For this review, take the finished solid that the model builds, in its own axes (mm). Round coordinates to 2 decimals unless told otherwise and drop trailing zeros. Loops run counter-clockwise (first coordinate to the right, second up) from the corner with the lowest first, then second, coordinate; pieces in that order, holes last.
1. Consider section D-D on z = 77. State the section outline as (x, y) points.
2. Consider section C-C on y = -16.5. State the section outline as (x, z) points.
3. Consider section A-A on z = 11. State the section outline as (x, y) points (3 decimals).
4. Consider section B-B on y = -162.5. State the section outline as (x, z) points, then the cut area to 3 significant figures.
5. Clearance check with flat-ended pins moving along their axes: pin 1 Ø5 at (y, z) = (-46.5, 99) entering from -X; pin 2 Ø0.9 at (x, y) = (2, -185.5) entering from +Z; pin 3 Ø0.9 at (x, y) = (1, -186) entering from -Z; pin 4 Ø0.9 at (x, z) = (1, 190.5) entering from +Y. State where each tip first meets the part, or that it passes through.
6. To check wall thickness, follow line 1 along Z through (x, y) = (1.7, -150); line 2 along Z through (x, y) = (1.4, -176); line 3 along Z through (x, y) = (0.35, -10). State the ranges of each line that lie inside material, in increasing order.
Autodesk Inventor part; units mm, degrees
ref_plane "YZ Plane" through (0, 0, 0) normal (1, 0, 0) x (0, 1, 0)
ref_plane "XZ Plane" through (0, 0, 0) normal (0, 1, 0) x (-1, 0, 0)
ref_plane "XY Plane" through (0, 0, 0) normal (0, 0, 1) x (1, 0, 0)
sketch "Sketch1" plane through (0, 0, 0) normal (1, 0, 0) x (0, 1, 0)
  line L0 (3, 191.4188) -> (-194, 191.4188) construction
  line L1 (-194, 191.4188) -> (-194, -8.5812) construction
  line L2 (-194, -8.5812) -> (3, -8.5812) construction
  line L3 (3, -8.5812) -> (3, 191.4188) construction
  line L4 (0, 188.4188) -> (-191, 188.4188) construction
  line L5 (-191, 188.4188) -> (-191, -5.5812) construction
  line L6 (-191, -5.5812) -> (0, -5.5812) construction
  line L7 (0, -5.5812) -> (0, 188.4188) construction
  line L8 (-165.5, -5.5812) -> (-165.5, -8.5812) construction
  line L9 (-194, -5.5812) -> (-165.5, -5.5812)
  line L10 (-165.5, -5.5812) -> (-165.5, -8.5812)
  line L11 (-165.5, -8.5812) -> (-145.5, -8.5812)
  line L12 (-145.5, -8.5812) -> (-145.5, -5.5812)
  line L13 (-145.5, -5.5812) -> (-125.5, -5.5812)
  line L14 (-125.5, -5.5812) -> (-125.5, -8.5812)
  line L15 (3, -5.5812) -> (-25.5, -5.5812)
  line L16 (-25.5, -5.5812) -> (-25.5, -8.5812)
  line L17 (-25.5, -8.5812) -> (-45.5, -8.5812)
  line L18 (-45.5, -8.5812) -> (-45.5, -5.5812)
  line L19 (-45.5, -5.5812) -> (-65.5, -5.5812)
  line L20 (-65.5, -5.5812) -> (-65.5, -8.5812)
  line L21 (-65.5, -8.5812) -> (-85.5, -8.5812)
  line L22 (-85.5, -8.5812) -> (-85.5, -5.5812)
  line L23 (-85.5, -5.5812) -> (-105.5, -5.5812)
  line L24 (-105.5, -5.5812) -> (-105.5, -8.5812)
  line L25 (-105.5, -8.5812) -> (-125.5, -8.5812)
  line L26 (-194, 188.4188) -> (-165.5, 188.4188)
  line L27 (-165.5, 188.4188) -> (-165.5, 191.4188)
  line L28 (3, 188.4188) -> (-25.5, 188.4188)
  line L29 (-25.5, 188.4188) -> (-25.5, 191.4188)
  line L30 (-25.5, 191.4188) -> (-45.5, 191.4188)
  line L31 (-45.5, 191.4188) -> (-45.5, 188.4188)
  line L32 (-45.5, 188.4188) -> (-65.5, 188.4188)
  line L33 (-65.5, 188.4188) -> (-65.5, 191.4188)
  line L34 (-65.5, 191.4188) -> (-85.5, 191.4188)
  line L35 (-85.5, 191.4188) -> (-85.5, 188.4188)
  line L36 (-85.5, 188.4188) -> (-105.5, 188.4188)
  line L37 (-105.5, 188.4188) -> (-105.5, 191.4188)
  line L38 (-105.5, 191.4188) -> (-125.5, 191.4188)
  line L39 (-125.5, 191.4188) -> (-125.5, 188.4188)
  line L40 (-125.5, 188.4188) -> (-145.5, 188.4188)
  line L41 (-145.5, 188.4188) -> (-145.5, 191.4188)
  line L42 (-145.5, 191.4188) -> (-165.5, 191.4188)
  line L43 (-194, 188.4188) -> (-194, 161.4188)
  line L44 (-194, 161.4188) -> (-191, 161.4188)
  line L45 (-191, 161.4188) -> (-191, 141.4188)
  line L46 (-191, 141.4188) -> (-194, 141.4188)
  line L47 (-194, 141.4188) -> (-194, 121.4188)
  line L48 (-194, 121.4188) -> (-191, 121.4188)
  line L49 (-194, -5.5812) -> (-194, 21.4188)
  line L50 (-194, 21.4188) -> (-191, 21.4188)
  line L51 (-191, 21.4188) -> (-191, 41.4188)
  line L52 (-191, 41.4188) -> (-194, 41.4188)
  line L53 (-194, 41.4188) -> (-194, 61.4188)
  line L54 (-194, 61.4188) -> (-191, 61.4188)
  line L55 (-191, 61.4188) -> (-191, 81.4188)
  line L56 (-191, 81.4188) -> (-194, 81.4188)
  line L57 (-194, 81.4188) -> (-194, 101.4188)
  line L58 (-194, 101.4188) -> (-191, 101.4188)
  line L59 (-191, 101.4188) -> (-191, 121.4188)
  line L60 (3, -5.5812) -> (3, 188.4188)
  line L61 (-194, 186.4008) -> (-146.985, 186.4008)
  line L62 (-146.985, 186.4008) -> (-146.985, 174.4008)
  line L63 (-177.985, 174.4008) -> (-177.985, 144.4008)
  line L64 (-177.985, 144.4008) -> (-165.985, 144.4008)
  line L65 (-165.985, 144.4008) -> (-165.985, 174.4008)
  line L66 (-194, -3.5632) -> (-146.985, -3.5632)
  line L67 (-146.985, -3.5632) -> (-146.985, 8.4368)
  line L68 (-146.985, 8.4368) -> (-165.985, 8.4368)
  line L69 (-165.985, 8.4368) -> (-165.985, 38.4368)
  line L70 (-165.985, 38.4368) -> (-177.985, 38.4368)
  line L71 (-177.985, 38.4368) -> (-177.985, 8.4368)
  line L72 (-177.985, 8.4368) -> (-194, 8.4368)
  line L73 (-177.985, 174.4008) -> (-194, 174.4008)
  line L74 (-146.985, 174.4008) -> (-165.985, 174.4008)
  point P0 (0, 0)
  point P1 (-170.4925, 186.4008)
  point P2 (-194, 174.9188)
  dimension "d0" = 197
  dimension "d1" = 200
  dimension "d2" = 3
  dimension "d3" = 3
  dimension "d4" = 3
  dimension "d5" = 3
  dimension "d6" = 3
  dimension "d7" = 3
  dimension "d8" = 3
  dimension "d9" = 3
  dimension "d11" = 28.5
  dimension "d12" = 20
  dimension "d13" = 20
  dimension "d14" = 28.5
  dimension "d15" = 20
  dimension "d16" = 20
  dimension "d17" = 20
  dimension "d18" = 20
  dimension "d19" = 28.5
  dimension "d20" = 28.5
  dimension "d21" = 20
  dimension "d22" = 20
  dimension "d23" = 20
  dimension "d24" = 20
  dimension "d25" = 20
  dimension "d26" = 20
  dimension "d27" = 27
  dimension "d28" = 20
  dimension "d29" = 20
  dimension "d30" = 27
  dimension "d31" = 20
  dimension "d32" = 20
  dimension "d33" = 20
  dimension "d34" = 20
  dimension "d35" = 5.018
  dimension "d37" = 47.015
  dimension "d38" = 12
  dimension "d39" = 19
  dimension "d40" = 30
  dimension "d41" = 12
  dimension "d42" = 16.015
  dimension "d43" = 5.018
  dimension "d47" = 47.015
  dimension "d48" = 30
  dimension "d49" = 12
  dimension "d50" = 12
  dimension "d51" = 19
  dimension "d52" = 16.015
extrude "Extrusion1" add sketch "Sketch1" along normal blind 3 contours L49 L66 L67 L68 L69 L70 L71 L72 L50 L51 L52 L53 L54 L55 L56 L57 L58 L59 L48 L47 L46 L45 L44 L43 L73 L63 L64 L65 L74 L62 L61 L26 L27 L42 L41 L40 L39 L38 L37 L36 L35 L34 L33 L32 L31 L30 L29 L28 L60 L15 L16 L17 L18 L19 L20 L21 L22 L23 L24 L25 L14 L13 L12 L11 L10 L9
sketch "Sketch2" plane through (3, 0, 0) normal (1, 0, 0) x (0, 0, -1)
  line L0 (5.5812, 3) -> (-188.4188, 3)
  line L1 (-135.4188, 3) -> (-47.4188, 3)
  line L2 (-47.4188, 3) -> (-47.4188, -47)
  line L3 (-47.4188, -47) -> (-135.4188, -47)
  line L4 (-135.4188, -47) -> (-135.4188, 3)
  point P0 (0, 0)
  dimension "d58" = 50
  dimension "d59" = 88
  dimension "d60" = 53
  dimension "d61" = 53
extrude "Extrusion2" cut sketch "Sketch2" against normal blind 10
properties part number "outisdewall_right"
Resolved:
1. outline: (0, -191) - (3, -191) - (3, -47) - (0, -47) - close
2. outline: (0, -5.58) - (3, -5.58) - (3, 47.42) - (0, 47.42) - close; (0, 135.42) - (3, 135.42) - (3, 188.42) - (0, 188.42) - close
3. outline: (0, -194) - (3, -194) - (3, -177.985) - (0, -177.985) - close; (0, -165.985) - (3, -165.985) - (3, 3) - (0, 3) - close
4. outline: (0, -8.58) - (3, -8.58) - (3, -3.56) - (0, -3.56) - close; (0, 8.44) - (3, 8.44) - (3, 174.4) - (0, 174.4) - close; (0, 186.4) - (3, 186.4) - (3, 191.42) - (0, 191.42) - close
4. area: 528 mm2
5. pin 1: stops at x = 0
5. pin 2: stops at z = 188.42
5. pin 3: stops at z = -5.58
5. pin 4: stops at y = -25.5
6. line 1: z = -8.58 to -3.56, 8.44 to 174.4, 186.4 to 191.42
6. line 2: z = -5.58 to -3.56, 38.44 to 144.4, 186.4 to 188.42
6. line 3: z = -5.58 to 47.42, 135.42 to 188.42
